Part model, mm, in its own coordinate system. A direction names the side the tool comes from. Round coordinates to 2 decimals unless told otherwise and drop trailing zeros. Order: outer loops, then holes, each group sorted by start corner. A loop starts at its lowest first (then second) coordinate and runs counter-clockwise, first axis right, second up. Notation, with made-up numbers: M -24,-24.5 L 29,-24.5 A16 cw 29,-9.5 Z; hole C -5,69.5 d2. An arc over 180 degrees is marked long. Write each question's results on one line, items separated by ' | '. Start each with the question number.
1. Band-saw the part on A-A, the plane z = 1. Give the number of separate pieces and of enclosed holes in the cut face, then the cut area to 3 significant figures.
2. Band-saw the part on C-C, the plane y = 10.5. List the corners of the cut face in (x, z) (3 decimals).
3. Two-plate mould, pull along X, no slides. Class faces 6 (the face through (57, -16, -9.525)), 7 (the face through (0, 5, 13)), 8 (the face through (13, -12.7, 28)), 9 (the face through (50.686, 25, 9)): +X half, -X half, draft (parallel to the pull), parting line (faces both ways), or undercut.
4. Band-saw the part on D-D, the plane z = 41. List the corners of the cut face in (x, y), then the cut area to 3 significant figures.
5. Band-saw the part on B-B, the plane x = 26. List the corners of the cut face in (y, z) (3 decimals).
6. Drop flat-ended pins along their axis: pin 1 Ø6.5 at (x, y) = (68.5, 17) entering from +Z (3 decimals); pin 2 Ø13 at (x, z) = (15, 31.5) entering from -Y; pin 3 Ø12 at (y, z) = (-14, 30) entering from +X. Give the stop position or say it passes through.
7. Probe L1, parallel to X at y = -4, z = 25; L2, parallel to Z at x = 37, y = 2; L3, parallel to Y at x = 73, z = -6.5. List the from-to ranges inside material, lowest first. Write a range as [from, to].
8. Which spindle directions (+Z, -Z, +X, -X, +Y, -Y) get a long thin tool onto all of the face, cutting with end or side? Do faces 1 (the face through (63.5, 19, 0)), 2 (the face through (70, -16, 9.525)), 3 (the face through (8, 0, 38.1)), 4 (the face through (24.988, 10.85, 31.578)), 5 (the face through (33.02, -10, 24)). Say none if no direction does.
```python
from build123d import *

# Parameters (mm, degrees)
F1_DEPTH = 50.8
F2_DEPTH = 63.5
F3_DEPTH = 33.02
F5_DEPTH = 50.801
F6_DEPTH = 50.8
F8_DEPTH = 12.7


with BuildPart() as f1:
    # F0 (on Right) → F1 (new body)
    with BuildSketch(Plane.YZ):
        with BuildLine():
            ThreePointArc((-8.4002604126, 9.525), (0, 12.7), (8.4002604126, 9.525))
            Line((8.4002604126, 9.525), (23.5464301965, 9.525))
            ThreePointArc((23.5464301965, 9.525), (8.2643354373, 24.017925801), (-12.7, 21.9970452561))
            ThreePointArc((-12.7, 21.9970452561), (-19.1660873346, 16.6679661712), (-23.5464301965, 9.525))
            Line((-23.5464301965, 9.525), (-8.4002604126, 9.525))
        make_face()
        with BuildLine():
            ThreePointArc((-8.4002604126, -9.525), (-12.7, 0), (-8.4002604126, 9.525))
            Line((-8.4002604126, 9.525), (-23.5464301965, 9.525))
            ThreePointArc((-23.5464301965, 9.525), (-25.4, 0), (-23.5464301965, -9.525))
            Line((-23.5464301965, -9.525), (-8.4002604126, -9.525))
        make_face()
    extrude(amount=F1_DEPTH)

    # F0 (on Right) → F2 (join)
    with BuildSketch(Plane.YZ):
        with BuildLine():
            Line((23.5464301965, -9.525), (8.4002604126, -9.525))
            ThreePointArc((8.4002604126, -9.525), (0, -12.7), (-8.4002604126, -9.525))
            Line((-8.4002604126, -9.525), (-23.5464301965, -9.525))
            ThreePointArc((-23.5464301965, -9.525), (0, -25.4), (23.5464301965, -9.525))
        make_face()
    extrude(amount=F2_DEPTH)

    # F0 (on Right) → F3 (join)
    with BuildSketch(Plane.YZ):
        with BuildLine():
            ThreePointArc((-12.7, 21.9970452561), (8.2643354373, 24.017925801), (23.5464301965, 9.525))
            ThreePointArc((23.5464301965, 9.525), (24.9323016085, 4.8518384664), (25.4, 0))
            Line((25.4, 0), (25.4, 50.8))
            Line((25.4, 50.8), (12.7, 50.8))
            Line((12.7, 50.8), (12.7, 38.1))
            Line((12.7, 38.1), (-12.7, 38.1))
            Line((-12.7, 38.1), (-12.7, 21.9970452561))
        make_face()
    extrude(amount=F3_DEPTH)

    # F4 (on face) → F5 (cut, through all)
    with BuildSketch(Plane(origin=(0, 25.4, 0), x_dir=(-1, 0, 0), z_dir=(0, 1, 0))):
        Polygon((-33.02, 50.8), (-33.02, 25.4), (0, 50.8), align=None)
    extrude(amount=-F5_DEPTH, mode=Mode.SUBTRACT)

    # F0 (on Right) → F6 (join)
    with BuildSketch(Plane.YZ):
        with BuildLine():
            Line((23.5464301965, -9.525), (8.4002604126, -9.525))
            ThreePointArc((8.4002604126, -9.525), (0, -12.7), (-8.4002604126, -9.525))
            Line((-8.4002604126, -9.525), (-23.5464301965, -9.525))
            ThreePointArc((-23.5464301965, -9.525), (0, -25.4), (23.5464301965, -9.525))
        make_face()
        with BuildLine():
            ThreePointArc((-8.4002604126, -9.525), (-12.7, 0), (-8.4002604126, 9.525))
            Line((-8.4002604126, 9.525), (-23.5464301965, 9.525))
            ThreePointArc((-23.5464301965, 9.525), (-25.4, 0), (-23.5464301965, -9.525))
            Line((-23.5464301965, -9.525), (-8.4002604126, -9.525))
        make_face()
        with BuildLine():
            ThreePointArc((8.4002604126, 9.525), (11.5752604126, 5.2252604126), (12.7, 0))
            ThreePointArc((12.7, 0), (11.5752604126, -5.2252604126), (8.4002604126, -9.525))
            Line((8.4002604126, -9.525), (23.5464301965, -9.525))
            ThreePointArc((23.5464301965, -9.525), (24.9323016085, -4.8518384664), (25.4, 0))
            ThreePointArc((25.4, 0), (24.9323016085, 4.8518384664), (23.5464301965, 9.525))
            Line((23.5464301965, 9.525), (8.4002604126, 9.525))
        make_face()
    extrude(amount=F6_DEPTH)

    # F7 (on face) → F8 (join)
    with BuildSketch(Plane.YZ.offset(63.5)):
        with BuildLine():
            Line((-8.4002604126, 9.525), (-23.5464301965, 9.525))
            ThreePointArc((-23.5464301965, 9.525), (-25.4, 0), (-23.5464301965, -9.525))
            Line((-23.5464301965, -9.525), (-8.4002604126, -9.525))
            ThreePointArc((-8.4002604126, -9.525), (-12.7, 0), (-8.4002604126, 9.525))
        make_face()
        with BuildLine():
            ThreePointArc((-23.5464301965, -9.525), (0, -25.4), (23.5464301965, -9.525))
            Line((23.5464301965, -9.525), (8.4002604126, -9.525))
            ThreePointArc((8.4002604126, -9.525), (0, -12.7), (-8.4002604126, -9.525))
            Line((-8.4002604126, -9.525), (-23.5464301965, -9.525))
        make_face()
        with BuildLine():
            ThreePointArc((23.5464301965, -9.525), (24.9323016085, -4.8518384664), (25.4, 0))
            ThreePointArc((25.4, 0), (24.9323016085, 4.8518384664), (23.5464301965, 9.525))
            Line((23.5464301965, 9.525), (8.4002604126, 9.525))
            ThreePointArc((8.4002604126, 9.525), (11.5752604126, 5.2252604126), (12.7, 0))
            ThreePointArc((12.7, 0), (11.5752604126, -5.2252604126), (8.4002604126, -9.525))
            Line((8.4002604126, -9.525), (23.5464301965, -9.525))
        make_face()
    extrude(amount=F8_DEPTH)

    # F9 (on face) → F10 (join, up to the next surface of F1)
    with BuildSketch(Plane(origin=(0, 25.4, 0), x_dir=(-1, 0, 0), z_dir=(0, 1, 0))):
        Polygon((-33.02, 0), (-33.02, 25.4), (-50.6857, 11.811), (-50.6857, 0), align=None)
    extrude(until=Until.NEXT, dir=(0, -1, 0))


solid = f1.part
```
Solution:
1) separate pieces: 4 | enclosed holes: 0 | area: 1,620 mm^2
2) outline: M 0,-23.128 L 76.2,-23.128 L 76.2,-7.144 L 63.5,-7.144 L 63.5,-9.525 L 50.8,-9.525 L 50.8,-7.144 L 0,-7.144 Z; M 0,7.144 L 50.8,7.144 L 50.8,23.128 L 35.973,23.128 L 16.51,38.1 L 0,38.1 Z; M 63.5,7.144 L 76.2,7.144 L 76.2,9.525 L 63.5,9.525 Z
3) face 6: undercut | face 7: -X half | face 8: draft | face 9: +X half
4) outline: M 0,12.7 L 12.74,12.7 L 12.74,25.4 L 0,25.4 Z | area: 162 mm^2
5) outline: M -12.7,21.997 A25.4 ccw long 25.4,0 L 25.4,30.8 L -12.7,30.8 Z; hole C 0,0 d25.4
6) pin 1: z = 9.525 | pin 2: y = -12.7 | pin 3: x = 33.02
7) L1: [0, 50.8] | L2: [-25.32, -12.54], [12.54, 25.32] | L3: [-24.55, -10.91], [10.91, 24.55]
8) face 1: +Z, +Y, -Y | face 2: +Z, +X, +Y, -Y | face 3: +Z, +X, -X, -Y | face 4: +Z, +X, +Y | face 5: +Z, +X, -Y
